Autodesk Inventor part; units mm, degrees
ref_plane "YZ Plane" through (0, 0, 0) normal (1, 0, 0) x (0, 1, 0)
ref_plane "XZ Plane" through (0, 0, 0) normal (0, 1, 0) x (-1, 0, 0)
ref_plane "XY Plane" through (0, 0, 0) normal (0, 0, 1) x (1, 0, 0)
sketch "Sketch1" plane through (0, 0, 0) normal (0, 1, 0) x (-1, 0, 0)
  line L0 (45, 22) -> (-45, 22)
  line L1 (-45, 22) -> (-45, -22)
  line L2 (-45, -22) -> (45, -22)
  line L3 (45, -22) -> (45, 22)
  line L4 (45, 22) -> (-45, -22) construction
  line L5 (-45, 22) -> (45, -22) construction
  point P0 (0, 0)
  dimension "d0" = 90
  dimension "d1" = 44
extrude "Extrusion1" add sketch "Sketch1" along normal blind 10
sketch "Sketch2" plane through (0, 10, 0) normal (0, 1, 0) x (1, 0, 0)
  line L0 (45, -22) -> (30, -22)
  line L1 (30, -22) -> (30, -17)
  line L2 (30, -17) -> (45, -17)
  line L3 (45, -17) -> (45, -22)
  line L4 (45, 17) -> (30, 17)
  line L5 (30, 17) -> (30, 22)
  line L6 (30, 22) -> (45, 22)
  line L7 (45, 22) -> (45, 17)
  line L8 (-45, -22) -> (-30, -22)
  line L9 (-30, -22) -> (-30, -17)
  line L10 (-30, -17) -> (-45, -17)
  line L11 (-45, -17) -> (-45, -22)
  line L12 (-45, 17) -> (-30, 17)
  line L13 (-30, 17) -> (-30, 22)
  line L14 (-30, 22) -> (-45, 22)
  line L15 (-45, 22) -> (-45, 17)
  line L16 (-45, 22) -> (-45, -22)
  line L17 (-45, -22) -> (45, -22)
  line L18 (45, 22) -> (-45, 22)
  line L19 (45, -22) -> (45, 22)
  point P0 (0, 0)
  dimension "d4" = 5
  dimension "d5" = 5
  dimension "d6" = 5
  dimension "d7" = 5
  dimension "d8" = 15
  dimension "d9" = 15
  dimension "d10" = 15
  dimension "d11" = 15
extrude "Extrusion2" add sketch "Sketch2" along normal blind 15 contours L0 L1 L2 L3 | L8 L11 L10 L9 | L4 L5 L6 L7 | L15 L14 L13 L12
sketch "Sketch3" plane through (-45, 0, 22) normal (0, 0, 1) x (1, 0, 0)
  circle A0 centre (82.5, 17.5) radius 2.05
  circle A1 centre (7.5, 17.5) radius 2.05
  line L0 (75, 25) -> (90, 25)
  line L1 (90, 0) -> (90, 25)
  line L2 (0, 25) -> (15, 25)
  line L3 (15, 10) -> (15, 25)
  point P0 (45, 0)
  point P1 (15, 17.5)
  dimension "d14" = 4.1
  dimension "d15" = 4.1
  dimension "d16" = 7.5
  dimension "d17" = 7.5
  dimension "d18" = 7.5
  dimension "d19" = 7.5
extrude "Extrusion3" cut sketch "Sketch3" against normal through all
sketch "Sketch4" plane through (0, 0, 0) normal (0, -1, 0) x (1, 0, 0)
  line L0 (-20, -22) -> (20, -22)
  line L1 (20, -22) -> (20, 22)
  line L2 (20, 22) -> (-20, 22)
  line L3 (-20, 22) -> (-20, -22)
  line L4 (-20, -22) -> (20, 22) construction
  line L5 (20, -22) -> (-20, 22) construction
  point P0 (0, 0)
  dimension "d22" = 40
  dimension "d23" = 44
extrude "Extrusion4" add sketch "Sketch4" along normal blind 4
sketch "Sketch5" plane through (0, -4, 0) normal (0, -1, 0) x (1, 0, 0)
  circle A0 centre (-12.5, -10) radius 1.55
  circle A1 centre (12.5, -10) radius 1.55
  circle A2 centre (-12.5, 10) radius 1.55
  circle A3 centre (12.5, 10) radius 1.55
  point P0 (0, 0)
  dimension "d26" = 3.1
  dimension "d27" = 3.1
  dimension "d28" = 3.1
  dimension "d29" = 3.1
  dimension "d30" = 12.5
  dimension "d31" = 12.5
  dimension "d32" = 12.5
  dimension "d33" = 12.5
  dimension "d34" = 10
  dimension "d35" = 10
  dimension "d36" = 10
  dimension "d37" = 10
extrude "Extrusion5" cut sketch "Sketch5" against normal through all
sketch "Sketch6" plane through (0, 10, 0) normal (0, 1, 0) x (1, 0, 0)
  circle A0 centre (12.5, -10) radius 1.55
  circle A1 centre (-12.5, -10) radius 1.55
  circle A2 centre (12.5, 10) radius 1.55
  circle A3 centre (-12.5, 10) radius 1.55
  circle A4 centre (12.5, -10) radius 5
  circle A5 centre (-12.5, -10) radius 5
  circle A6 centre (12.5, 10) radius 5
  circle A7 centre (-12.5, 10) radius 5
  point P0 (0, 0)
  dimension "d40" = 10
  dimension "d41" = 10
  dimension "d42" = 10
  dimension "d43" = 10
extrude "Extrusion6" cut sketch "Sketch6" against normal blind 7
properties part number "rail_top" material "ABS Plastic"
Here's how the part is built. I have some questions about the finished solid (model axes, mm). A direction names the side the tool comes from. Give positions to 0.01 mm unless a question says otherwise; leave off trailing zeros. Loops run counter-clockwise (first coordinate to the right, second up) from the corner with the lowest first, then second, coordinate; pieces in that order, holes last. Notation, with made-up numbers: M 47,-17.5 L 93,-17.5 A20 cw 93,-2.5 Z; hole C -40,35 d2. An arc over 180 degrees is marked long. Put each result on its own line as item: value. Start each with the question number.
(1) I want a section at D-D on y = 13.5. Please give me the cut outline in (x, z).
(2) I need wall thicknesses on line 1 along Z through (x, y) = (12.5, -2.5); line 2 along Z through (x, y) = (12.5, 7); line 3 along Y through (x, z) = (-37.5, 20.1). Which ranges of each line are inside material? Lowest first, please. Write a range as [from, to].
(3) I want a section at A-A on y = 17.5. State how many separate pieces and enclosed holes the cut face has, then the cut area to 3 significant figures.
(4) Will these pins go through, and if not, where does the flat tip stop? pin 1 Ø16 at (x, z) = (-12.5, 10) entering from -Y; pin 2 Ø11 at (x, z) = (-13.5, 12) entering from +Y; pin 3 Ø4 at (x, z) = (12.5, -10) entering from +Y.
(5) For faces 1 (the flat face through (33, 0, 0)), 2 (the flat face through (-14, 3, 11)), 3 (the flat face through (30, 17, -19)), 4 (the flat face through (39.3, 15.7, -17)), which set-ups out of +Z, -Z, +X, -X, +Y, -Y let a thin tool reach every point of the face, with its end or its side?
(6) I want a section at C-C on z = 10. Please give me the cut outline in (x, y).
(7) I want a section at B-B on x = -37.5. Please give me the cut outline in (y, z), then the cut area to 3 significant figures.
(8) If we mould it in two halves opening along X, with no side actions, what happens to faces 5 (the flat face through (20, -2, 0)), 6 (the cylindrical face through (11.27, -0.55, -10.94)), 7 (the flat face through (-39.3, 15.7, -17))? For each: +X half, -X half, draft (parallel to the pull), parting line (faces both ways), or undercut.
Answer block:
1. outline: M -45,-22 L -30,-22 L -30,-17 L -45,-17 Z; M -45,17 L -30,17 L -30,22 L -45,22 Z; M 30,-22 L 45,-22 L 45,-17 L 30,-17 Z; M 30,17 L 45,17 L 45,22 L 30,22 Z
2. line 1: [-22, -11.55], [-8.45, 8.45], [11.55, 22]
2. line 2: [-22, -15], [-5, 5], [15, 22]
2. line 3: [0, 15.45], [19.55, 25]
3. separate pieces: 8
3. enclosed holes: 0
3. area: 218 mm^2
4. pin 1: y = -4
4. pin 2: y = 10
4. pin 3: y = 3
5. face 1: +Z, -Z, +X, -Y
5. face 2: +Y
5. face 3: +Z, -Z, +Y
5. face 4: +X, -X, +Y
6. outline: M -45,0 L -20,0 L -20,-4 L -14.05,-4 L -14.05,3 L -17.5,3 L -17.5,10 L -45,10 Z; M -10.95,-4 L 10.95,-4 L 10.95,3 L 7.5,3 L 7.5,10 L -7.5,10 L -7.5,3 L -10.95,3 Z; M 14.05,-4 L 20,-4 L 20,0 L 45,0 L 45,10 L 17.5,10 L 17.5,3 L 14.05,3 Z
7. outline: M 0,-22 L 15.45,-22 L 15.45,-17 L 10,-17 L 10,17 L 15.45,17 L 15.45,22 L 0,22 Z; M 19.55,-22 L 25,-22 L 25,-17 L 19.55,-17 Z; M 19.55,17 L 25,17 L 25,22 L 19.55,22 Z
7. area: 549 mm^2
8. face 5: +X half
8. face 6: undercut
8. face 7: draft
